Check sheet for the modelled part. Datum: model origin and axes. Units: mm. Face numbers are marked on the shaded views. A direction names the side the tool comes from. Give positions to 0.01 mm unless a question says otherwise; leave off trailing zeros. Loops run counter-clockwise (first coordinate to the right, second up) from the corner with the lowest first, then second, coordinate; pieces in that order, holes last. Notation, with made-up numbers: (54.25, 83.25) - (87.25, 83.25) arc R21 ccw to (87.25, 89.25) - close; hole circle Ø5 at (40.25, 74.25). An arc over 180 degrees is marked (long way). Use one line per item in the form item = value.
from build123d import *

# Parameters (mm, degrees)
ESQUISSE1_R             = 44.8
ESQUISSE1_R_2           = 10.15
ESQUISSE1_R_3           = 1.8
BOSS_EXTRU_1_DEPTH      = 7
BOSS_EXTRU_2_START      = 3
ESQUISSE3_R             = 44.8
ESQUISSE3_R_2           = 33.5
BOSS_EXTRU_2_DEPTH      = 3
ESQUISSE4_R             = 2.85
ENL_V_MAT_EXTRU_3_DEPTH = 3.7


with BuildPart() as part:
    # Esquisse1 → Boss.-Extru.1 (new body)
    with BuildSketch(Plane.XY):
        Circle(ESQUISSE1_R)
        with Locations((-10.25, 0)):
            Circle(ESQUISSE1_R_2, mode=Mode.SUBTRACT)
        with Locations((0, 30)):
            Circle(ESQUISSE1_R_3, mode=Mode.SUBTRACT)
        with Locations(Location((0, -30, 0), (0, 0, 180))):
            Circle(ESQUISSE1_R_3, mode=Mode.SUBTRACT)
    extrude(amount=BOSS_EXTRU_1_DEPTH)

    # Esquisse3 → Boss.-Extru.2 (add)
    with BuildSketch(Plane(origin=(0, 0, 0), x_dir=(-1, 0, 0), z_dir=(0, 0, -1)).offset(BOSS_EXTRU_2_START)):
        Circle(ESQUISSE3_R)
        Circle(ESQUISSE3_R_2, mode=Mode.SUBTRACT)
    extrude(amount=-BOSS_EXTRU_2_DEPTH)

    # Esquisse4 → Enlèv. mat.-Extru.3 (cut)
    with BuildSketch(Plane.XY.offset(7)):
        with Locations((0, 30)):
            Circle(ESQUISSE4_R)
        with Locations((0, -30)):
            Circle(ESQUISSE4_R)
    extrude(amount=-ENL_V_MAT_EXTRU_3_DEPTH, mode=Mode.SUBTRACT)


solid = part.part
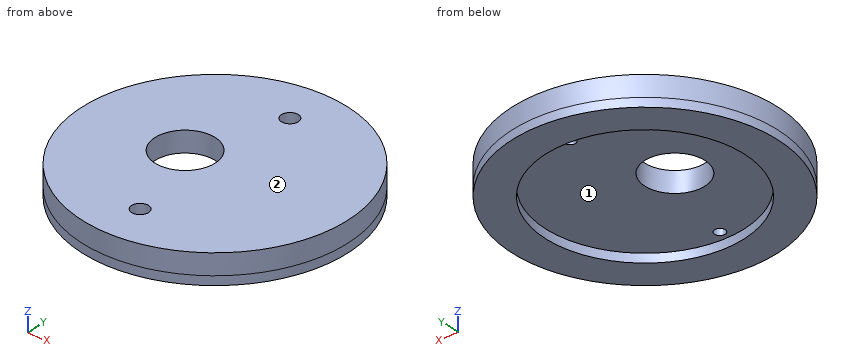
Item 1: Gauge pin test, flat ends, axial feed: P1, Ø6, axis at y = -24, z = -1.5, coming from the -X side; P2, Ø1.5, axis at x = 24.5, z = -0.5, coming from the -Y side; P3, Ø4.5, axis at x = 0, y = -30, coming from the +Z side; P4, Ø3, axis at x = 1, y = 28.5, coming from the +Z side. Record the tip position at first contact, or that the pin passes through.
Answer block:
P1 = -39.57
P2 = -37.99
P3 = 3.3
P4 = 7
Item 2: Section check B-B on z = 5.75. Record the boundary of the cut face in (x, y), then the cut area to 3 significant figures.
Answer block:
outline = circle Ø89.6 at (0, 0); hole circle Ø20.3 at (-10.25, 0); hole circle Ø5.7 at (0, -30); hole circle Ø5.7 at (0, 30)
area = 5,930 mm2
Item 3: Section check A-A on y = 0. Record the boundary of the cut face in (x, z), then the cut area to 3 significant figures.
Answer block:
outline = (-44.8, -3) - (-33.5, -3) - (-33.5, 0) - (-20.4, 0) - (-20.4, 7) - (-44.8, 7) - close; (-0.1, 0) - (33.5, 0) - (33.5, -3) - (44.8, -3) - (44.8, 7) - (-0.1, 7) - close
area = 553 mm2
Item 4: Section check C-C on x = -10.25. Record the boundary of the cut face in (y, z).
Answer block:
outline = (-43.61, -3) - (-31.89, -3) - (-31.89, 0) - (-10.15, 0) - (-10.15, 7) - (-43.61, 7) - close; (10.15, 0) - (31.89, 0) - (31.89, -3) - (43.61, -3) - (43.61, 7) - (10.15, 7) - close
Item 5: Thickness scan on L1, parallel to Y at x = 0, z = 6.1; L2, parallel to Y at x = 0, z = 1.35; L3, parallel to Y at x = 0.5, z = -0.25. Record the ranges inside material, lowest first.
Answer block:
L1 = -44.8 to -32.85, -27.15 to 27.15, 32.85 to 44.8
L2 = -44.8 to -31.8, -28.2 to 28.2, 31.8 to 44.8
L3 = -44.8 to -33.5, 33.5 to 44.8
Item 6: Access from +Z, -Z, +X, -X, +Y, -Y to the whole of each face (thin tool, end or side, straight path). Record for the marked faces 1 and 2.
Answer block:
face_1 = -Z
face_2 = +Z, +X, -X, +Y, -Y
Item 7: Section check D-D on y = 30. Record the boundary of the cut face in (x, z), then the cut area to 3 significant figures.
Answer block:
outline = (-33.27, -3) - (-14.91, -3) - (-14.91, 0) - (-1.8, 0) - (-1.8, 3.3) - (-2.85, 3.3) - (-2.85, 7) - (-33.27, 7) - close; (1.8, 0) - (14.91, 0) - (14.91, -3) - (33.27, -3) - (33.27, 7) - (2.85, 7) - (2.85, 3.3) - (1.8, 3.3) - close
area = 543 mm2
